from build123d import *

# Parameters (mm, degrees)
SKETCH1_R           = 60
SKETCH1_R_2         = 2
BOSS_EXTRUDE1_DEPTH = 10
SKETCH2_R           = 60
SKETCH2_R_2         = 46
BOSS_EXTRUDE2_DEPTH = 35


with BuildPart() as part:
    # Sketch1 → Boss-Extrude1 (new body)
    with BuildSketch(Plane(origin=(0, 0, 0), x_dir=(1, 0, 0), z_dir=(0, 1, 0))):
        with Locations(Location((0, 0, 0), (0, 0, 270))):
            Circle(SKETCH1_R)
        with Locations(Location((0, 28, 0), (0, 0, 270))):
            Circle(SKETCH1_R_2, mode=Mode.SUBTRACT)
        with Locations(Location((24.248711306, 14, 0), (0, 0, 270))):
            Circle(SKETCH1_R_2, mode=Mode.SUBTRACT)
        with Locations(Location((24.248711306, -14, 0), (0, 0, 270))):
            Circle(SKETCH1_R_2, mode=Mode.SUBTRACT)
        with Locations(Location((0, -28, 0), (0, 0, 270))):
            Circle(SKETCH1_R_2, mode=Mode.SUBTRACT)
        with Locations(Location((-24.248711306, -14, 0), (0, 0, 270))):
            Circle(SKETCH1_R_2, mode=Mode.SUBTRACT)
        with Locations(Location((-24.248711306, 14, 0), (0, 0, 270))):
            Circle(SKETCH1_R_2, mode=Mode.SUBTRACT)
    extrude(amount=BOSS_EXTRUDE1_DEPTH)

    # Sketch2 → Boss-Extrude2 (add)
    with BuildSketch(Plane(origin=(0, 10, 0), x_dir=(1, 0, 0), z_dir=(0, 1, 0))):
        with Locations(Location((0, 0, 0), (0, 0, 270))):
            Circle(SKETCH2_R)
        with Locations(Location((0, 0, 0), (0, 0, 270))):
            Circle(SKETCH2_R_2, mode=Mode.SUBTRACT)
    extrude(amount=BOSS_EXTRUDE2_DEPTH)


solid = part.part
The listing builds one solid part. Answer for the finished solid, in the listing's coordinates (mm). A direction names the side the tool comes from. Give positions to 0.01 mm unless a question says otherwise; leave off trailing zeros. Write each loop counter-clockwise with the first axis right and the second up, starting at its lowest first coordinate (ties: lowest second). Pieces come first, ordered by that corner, then holes. Notation, with made-up numbers: (5.25, -0.75) -> (35.25, -0.75) arc R20 cw to (35.25, 10.25) -> close; hole circle Ø10 at (36.25, 36). An arc over 180 degrees is marked (long way). Use a Markdown table: item, result.
(1) Find the intervals of material crossed by probe 1 along Z at (x, y) = (-23, 4); probe 2 along Y at (x, z) = (-16.5, -37); probe 3 along X at (y, z) = (24, 0), in increasing order. Write a range as from..to.
Return value:
| item | result |
|---|---|
| probe 1 | -55.42..-15.56, -12.44..12.44, 15.56..55.42 |
| probe 2 | 0..10 |
| probe 3 | -60..-46, 46..60 |
(2) Section C-C, the plane y = 5.5 is taken. Determine the outline of the cut face in (x, z).
Return value:
| item | result |
|---|---|
| outline | circle Ø120 at (0, 0); hole circle Ø4 at (-24.25, -14); hole circle Ø4 at (-24.25, 14); hole circle Ø4 at (0, -28); hole circle Ø4 at (0, 28); hole circle Ø4 at (24.25, -14); hole circle Ø4 at (24.25, 14) |
(3) For faces 1 (the cylindrical face through (-0.766, 4.93, 29.847)), 2 (the flat face through (1, 10, -1)), determine the directions among +Z, -Z, +X, -X, +Y, -Y from which every point of the face is accessible in a straight line to the end or side of a thin tool.
Return value:
| item | result |
|---|---|
| face 1 | +Y, -Y |
| face 2 | +Y |
(4) Flat-ended cylindrical pins translate along their axes: P1, Ø6.5, axis at x = -24.25, z = 14, coming from the +Y side; P2, Ø12, axis at x = 36.5, y = 5, coming from the +Z side; P3, Ø4, axis at y = 7.5, z = -26, coming from the +X side. Find the tip coordinate at first contact, or state that the pin passes through.
Return value:
| item | result |
|---|---|
| P1 | y = 10 |
| P2 | z = 51.67 |
| P3 | x = 54.99 |
(5) Section A-A, the plane x = 0 is taken. Determine the outline of the cut face in (y, z), then the cut area to 3 significant figures.
Return value:
| item | result |
|---|---|
| outline | (0, -60) -> (45, -60) -> (45, -46) -> (10, -46) -> (10, -30) -> (0, -30) -> close; (0, -26) -> (10, -26) -> (10, 26) -> (0, 26) -> close; (0, 30) -> (10, 30) -> (10, 46) -> (45, 46) -> (45, 60) -> (0, 60) -> close |
| area | 2,100 mm2 |
(6) Section B-B, the plane z = 14 is taken. Determine the outline of the cut face in (x, y).
Return value:
| item | result |
|---|---|
| outline | (-58.34, 0) -> (-26.25, 0) -> (-26.25, 10) -> (-43.82, 10) -> (-43.82, 45) -> (-58.34, 45) -> close; (-22.25, 0) -> (22.25, 0) -> (22.25, 10) -> (-22.25, 10) -> close; (26.25, 0) -> (58.34, 0) -> (58.34, 45) -> (43.82, 45) -> (43.82, 10) -> (26.25, 10) -> close |
(7) Determine the mould class of faces 3 (the cylindrical face through (2.64, 22.18, -59.94)), 4 (the cylindrical face through (38.787, 27.255, 24.729)), 5 (the flat face through (1, 0, -1)) for opening direction X: released by +X, released by -X, zero draft, split by the parting line, or undercut.
Return value:
| item | result |
|---|---|
| face 3 | split by the parting line |
| face 4 | undercut |
| face 5 | zero draft |
(8) Section D-D, the plane z = 28 is taken. Determine the outline of the cut face in (x, y).
Return value:
| item | result |
|---|---|
| outline | (-53.07, 0) -> (-2, 0) -> (-2, 10) -> (-36.5, 10) -> (-36.5, 45) -> (-53.07, 45) -> close; (2, 0) -> (53.07, 0) -> (53.07, 45) -> (36.5, 45) -> (36.5, 10) -> (2, 10) -> close |
